Part model, mm, in its own coordinate system. Face numbers are marked on the shaded views. A direction names the side the tool comes from. Round coordinates to 2 decimals unless told otherwise and drop trailing zeros. Write each loop counter-clockwise with the first axis right and the second up, starting at its lowest first coordinate (ties: lowest second). Pieces come first, ordered by that corner, then holes. Notation, with made-up numbers: (51.5, 28) -> (61.5, 28) arc R17 cw to (61.5, 36) -> close; hole circle Ø8 at (1, 51). An arc over 180 degrees is marked (long way). Use CSV: the item, a comma, the result in double quotes. Start each with the question number.
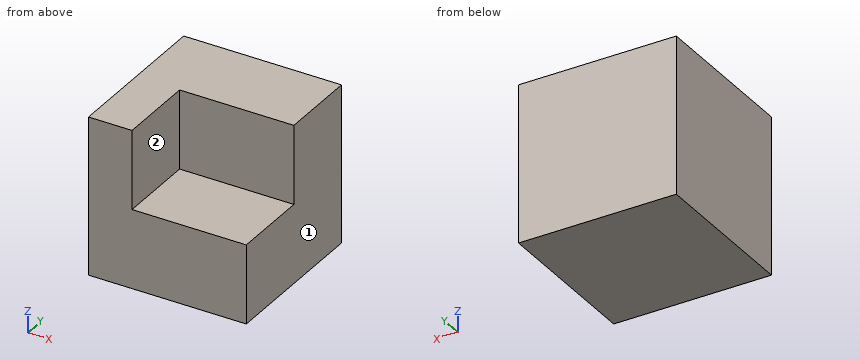
```python
from build123d import *

# Parameters (mm, degrees)
F1_DEPTH = 50.8
F2_W     = 36.796042
F2_H     = 25.4
F3_DEPTH = 25.4


with BuildPart() as f1:
    # F0 (on Front) → F1 (new body)
    with BuildSketch(Plane.XZ):
        Polygon((-51.370482, -39.115857), (-0.570482, -39.115857), (-0.570482, -13.715857), (-37.366524, -13.715857), (-37.366524, 11.684143), (-51.370482, 11.684143), align=None)
    extrude(amount=F1_DEPTH)

    # F2 (on face) → F3 (join)
    with BuildSketch(Plane.XY.offset(-13.715857)):
        with Locations((-18.968503, -12.7)):
            Rectangle(F2_W, F2_H)
    extrude(amount=F3_DEPTH)


solid = f1.part
```
1. Flat gauge pins, fed straight in: pin 1 (1.5 mm diameter, centred on x = -27.5, y = -26.5, fed in from +Z); pin 2 (2 mm diameter, centred on x = -30, z = 3, fed in from -Y); pin 3 (12 mm diameter, centred on x = -18, z = -32.5, fed in from +Y). Where does each tip first touch, or does it go through?
2. Band-saw the part on A-A (x = -27.5). List the corners of the cut face in (y, z).
3. Drill centre lines: line 1 along Z through (x, y) = (-9.5, -39); line 2 along Y through (x, z) = (-24, 5.5); line 3 along X through (y, z) = (-27, 6). Where is each one in solid material? Low to high. Write a range as [from, to].
4. Which spindle directions (+Z, -Z, +X, -X, +Y, -Y) get a long thin tool onto all of the face, cutting with end or side? Do the marked faces 1 and 2. Say none if no direction does.
5. Band-saw the part on B-B (y = -41). List the corners of the cut face in (x, z).
Answers below:
1,pin 1,"stops at z = -13.72"
1,pin 2,"stops at y = -25.4"
1,pin 3,"stops at y = 0"
2,outline,"(-50.8, -39.12) -> (0, -39.12) -> (0, 11.68) -> (-25.4, 11.68) -> (-25.4, -13.72) -> (-50.8, -13.72) -> close"
3,line 1,"z = [-39.12, -13.72]"
3,line 2,"y = [-25.4, 0]"
3,line 3,"x = [-51.37, -37.37]"
4,face 1,"+Z, -Z, +X, +Y, -Y"
4,face 2,"+Z, +X, -Y"
5,outline,"(-51.37, -39.12) -> (-0.57, -39.12) -> (-0.57, -13.72) -> (-37.37, -13.72) -> (-37.37, 11.68) -> (-51.37, 11.68) -> close"
